```python
from build123d import *

# Parameters (mm, degrees)
BOSS_EXTRUDE1_DEPTH      = 7
EXTRUDE_THIN2_DEPTH      = 15
FILLET1_R                = 7
SKETCH5_W                = 15
SKETCH5_H                = 25
BOSS_EXTRUDE2_DEPTH      = 8
CUT_EXTRUDE2_DEPTH       = 42.641325627
LPATTERN1_COUNT          = 2
LPATTERN1_PITCH          = 26
CHAMFER3_SIZE            = 7
SKETCH9_W                = 15
SKETCH9_H                = 7
BOSS_EXTRUDE3_DEPTH      = 15
BOSS_EXTRUDE4_DEPTH      = 2
BOSS_EXTRUDE4_DEPTH_BACK = 9.9
SKETCH13_W               = 8
SKETCH13_H               = 2
BOSS_EXTRUDE6_DEPTH      = 6
CHAMFER6_SIZE            = 23.744712882
CHAMFER6_SIZE_2          = 13.5
CHAMFER7_SIZE            = 3
SKETCH14_R               = 1.5
CUT_EXTRUDE3_DEPTH       = 15
SKETCH15_W               = 15
SKETCH15_H               = 8.5
CUT_EXTRUDE4_DEPTH       = 6
CHAMFER8_SIZE            = 8
SKETCH16_W               = 3
SKETCH16_H               = 20
CUT_EXTRUDE5_DEPTH       = 54.176035971


with BuildPart() as part:
    # Sketch1 → Boss-Extrude1 (new body)
    with BuildSketch(Plane.XY):
        with BuildLine():
            Line((0, 25), (-20, 25))
            Line((-20, 25), (-20, -25))
            Line((-20, -25), (25, -25))
            Line((25, -25), (25, 0))
            ThreePointArc((25, 0), (17.67766953, 17.67766953), (0, 25))
        make_face()
    extrude(amount=BOSS_EXTRUDE1_DEPTH)

    # Sketch3 → Extrude-Thin2 (add)
    with BuildSketch(Plane.XY.offset(7)):
        with BuildLine():
            Line((25, -25), (25, 0))
            ThreePointArc((25, 0), (17.67766953, 17.67766953), (0, 25))
            Line((0, 25), (-20, 25))
            Line((-20, 25), (-20, 21))
            Line((-20, 21), (0, 21))
            ThreePointArc((0, 21), (14.849242405, 14.849242405), (21, 0))
            Line((21, 0), (21, -25))
            Line((21, -25), (25, -25))
        make_face()
    extrude(amount=EXTRUDE_THIN2_DEPTH)

    # Fillet1
    fillet1_edges = [part.edges().sort_by_distance(p)[0] for p in [
        (21, -12.5, 7),
        (14.849242405, 14.849242405, 7),
        (-10, 21, 7),
    ]]
    fillet(fillet1_edges, radius=FILLET1_R)

    # Sketch5 → Boss-Extrude2 (add)
    with BuildSketch(Plane(origin=(25, 0, 0), x_dir=(0, 0, -1), z_dir=(1, 0, 0))):
        with Locations((7.5, -12.5)):
            Rectangle(SKETCH5_W, SKETCH5_H)
    extrude(amount=-BOSS_EXTRUDE2_DEPTH)

    # Sketch8 → Cut-Extrude2 (cut, through all)
    with BuildSketch(Plane.XY.offset(7)):
        with BuildLine():
            Line((-14, -15), (-2, -15))
            ThreePointArc((-2, -15), (0, -17), (-2, -19))
            Line((-2, -19), (-14, -19))
            ThreePointArc((-14, -19), (-16, -17), (-14, -15))
        make_face()
    cut_extrude2 = extrude(amount=-CUT_EXTRUDE2_DEPTH, mode=Mode.SUBTRACT)

    # LPattern1: Cut-Extrude2 ×2
    with Locations(*[(0, i * LPATTERN1_PITCH, 0) for i in range(1, LPATTERN1_COUNT)]):
        add(cut_extrude2, mode=Mode.SUBTRACT)

    # Chamfer3
    chamfer3_edges = [part.edges().sort_by_distance(p)[0] for p in [
        (25, -12.5, -15),
    ]]
    chamfer(chamfer3_edges, length=CHAMFER3_SIZE)

    # Sketch9 → Boss-Extrude3 (add)
    with BuildSketch(Plane.ZY.offset(-17)):
        with Locations((-7.5, -3.5)):
            Rectangle(SKETCH9_W, SKETCH9_H)
    extrude(amount=BOSS_EXTRUDE3_DEPTH)

    # Sketch10 → Boss-Extrude4 (add, two sides: drawn at the far end of the back side and taken through both)
    with BuildSketch(Plane.XZ.offset(7).offset(-BOSS_EXTRUDE4_DEPTH_BACK)):
        Polygon((2, -15), (-6.970562748, -15), (-12.627416998, -9.343145751), (-16.870057685, -13.585786438), (-20, -10.455844123), (-20, 0), (17, 0), (17, -15), align=None)
        Polygon((-4.849242405, -10.050252532), (-9.091883092, -5.807611845), (-6.970562748, -3.686291501), (-2.727922061, -7.928932188), align=None, mode=Mode.SUBTRACT)
    extrude(amount=BOSS_EXTRUDE4_DEPTH + BOSS_EXTRUDE4_DEPTH_BACK)

    # Sketch13 → Boss-Extrude6 (add)
    with BuildSketch(Plane(origin=(-10.985281374, 0, -10.985281374), x_dir=(-0.7071067811865478, 0, 0.7071067811865472), z_dir=(-0.7071067811865472, 0, -0.7071067811865478))):
        with Locations((-1.67766953, 1.9)):
            Rectangle(SKETCH13_W, SKETCH13_H)
        with Locations((-1.67766953, -8)):
            Rectangle(SKETCH13_W, SKETCH13_H)
    extrude(amount=BOSS_EXTRUDE6_DEPTH)

    # Chamfer6
    # the kernel refuses this chamfer: 23.744712882, 13.5 mm, written as the material it adds along each edge
    with BuildSketch(Plane(origin=(-6.970562748, -9, -15), x_dir=(-0.7145740403020574, 0, -0.6995598194053126), z_dir=(0, 1, 0))) as chamfer6_piece_1_section:
        Polygon((CHAMFER6_SIZE * 0.999943641689, -CHAMFER6_SIZE * 0.0106166574102), (-CHAMFER6_SIZE_2 * 0.714574040302, -CHAMFER6_SIZE_2 * 0.699559819405), (0, 0), align=None)
    chamfer6_piece_1 = extrude(amount=2, mode=Mode.PRIVATE)
    chamfer6_piece_1 = split(chamfer6_piece_1, bisect_by=Plane(origin=(-9.095447466, -8, -21.360396657), z_dir=(0.7071067811865476, 0, 0.7071067811865476)), keep=Keep.TOP, mode=Mode.PRIVATE)
    add(chamfer6_piece_1)
    with BuildSketch(Plane(origin=(-6.970562748, -70.647744863, -15), x_dir=(-0.7145740403020574, 0, -0.6995598194053126), z_dir=(0, 1, 0))) as chamfer6_piece_2_section:
        Polygon((CHAMFER6_SIZE * 0.999943641689, -CHAMFER6_SIZE * 0.0106166574102), (-CHAMFER6_SIZE_2 * 0.714574040302, -CHAMFER6_SIZE_2 * 0.699559819405), (0, 0), align=None)
    chamfer6_piece_2 = extrude(amount=125.295489727, mode=Mode.PRIVATE)
    chamfer6_piece_2 = split(chamfer6_piece_2, bisect_by=Plane(origin=(-6.871868761, 2.9, -19.136817952), z_dir=(0, -1, 0)), keep=Keep.TOP, mode=Mode.PRIVATE)
    chamfer6_piece_2 = split(chamfer6_piece_2, bisect_by=Plane(origin=(-6.871868761, 0.9, -19.136817952), z_dir=(0, 1, 0)), keep=Keep.TOP, mode=Mode.PRIVATE)
    chamfer6_piece_2 = split(chamfer6_piece_2, bisect_by=Plane(origin=(-9.095447466, 1.9, -21.360396657), z_dir=(0.7071067811865476, 0, 0.7071067811865476)), keep=Keep.TOP, mode=Mode.PRIVATE)
    add(chamfer6_piece_2)
    with BuildSketch(Plane(origin=(-6.970562748, -60.747744863, -15), x_dir=(-0.7145740403020574, 0, -0.6995598194053126), z_dir=(0, 1, 0))) as chamfer6_piece_3_section:
        Polygon((CHAMFER6_SIZE * 0.999943641689, -CHAMFER6_SIZE * 0.0106166574102), (-CHAMFER6_SIZE_2 * 0.714574040302, -CHAMFER6_SIZE_2 * 0.699559819405), (0, 0), align=None)
    chamfer6_piece_3 = extrude(amount=125.295489727, mode=Mode.PRIVATE)
    chamfer6_piece_3 = split(chamfer6_piece_3, bisect_by=Plane(origin=(-6.871868761, -7, -19.136817952), z_dir=(0, -1, 0)), keep=Keep.TOP, mode=Mode.PRIVATE)
    chamfer6_piece_3 = split(chamfer6_piece_3, bisect_by=Plane(origin=(-9.095447466, -8, -21.360396657), z_dir=(0.7071067811865476, 0, 0.7071067811865476)), keep=Keep.TOP, mode=Mode.PRIVATE)
    chamfer6_piece_3 = split(chamfer6_piece_3, bisect_by=Plane(origin=(-6.871868761, -9, -19.136817952), z_dir=(0, 1, 0)), keep=Keep.TOP, mode=Mode.PRIVATE)
    add(chamfer6_piece_3)
    with BuildSketch(Plane(origin=(-6.970562748, 0.9, -15), x_dir=(-0.7145740403020574, 0, -0.6995598194053126), z_dir=(0, 1, 0))) as chamfer6_piece_4_section:
        Polygon((CHAMFER6_SIZE * 0.999943641689, -CHAMFER6_SIZE * 0.0106166574102), (-CHAMFER6_SIZE_2 * 0.714574040302, -CHAMFER6_SIZE_2 * 0.699559819405), (0, 0), align=None)
    chamfer6_piece_4 = extrude(amount=2, mode=Mode.PRIVATE)
    chamfer6_piece_4 = split(chamfer6_piece_4, bisect_by=Plane(origin=(-9.095447466, 1.9, -21.360396657), z_dir=(0.7071067811865476, 0, 0.7071067811865476)), keep=Keep.TOP, mode=Mode.PRIVATE)
    add(chamfer6_piece_4)

    # Chamfer7
    chamfer7_edges = [part.edges().sort_by_distance(p)[0] for p in [
        (-1.5, 2.9, 0),
        (17, -9, -7.5),
        (17, -17, 0),
        (-1.5, -9, 0),
    ]]
    chamfer(chamfer7_edges, length=CHAMFER7_SIZE)

    # Sketch14 → Cut-Extrude3 (cut)
    with BuildSketch(Plane(origin=(-10.985281374, 0, -10.985281374), x_dir=(-0.7071067811865478, 0, 0.7071067811865472), z_dir=(-0.7071067811865472, 0, -0.7071067811865478))):
        with Locations((-0.67766953, -3.05)):
            Circle(SKETCH14_R)
    extrude(amount=-CUT_EXTRUDE3_DEPTH, mode=Mode.SUBTRACT)

    # Sketch15 → Cut-Extrude4 (cut)
    with BuildSketch(Plane(origin=(-15.227922061, 0, -15.227922061), x_dir=(-0.7071067811865475, 0, 0.7071067811865477), z_dir=(-0.7071067811865477, 0, -0.7071067811865475))):
        with Locations((-4.87766953, -3.05)):
            Rectangle(SKETCH15_W, SKETCH15_H)
    extrude(amount=-CUT_EXTRUDE4_DEPTH, mode=Mode.SUBTRACT)

    # Chamfer8
    # the kernel refuses this chamfer: 8 mm, written as the material it adds along each edge
    with BuildSketch(Plane(origin=(17, 0, 0), x_dir=(0.9996219169112968, -0.02749587661058649, 0), z_dir=(0, 0, -1))) as chamfer8_piece_1_section:
        Polygon((CHAMFER8_SIZE * 0.999621916911, -CHAMFER8_SIZE * 0.0274958766106), (-CHAMFER8_SIZE * 0.0274958766106, -CHAMFER8_SIZE * 0.999621916911), (0, 0), align=None)
    chamfer8_piece_1 = extrude(amount=15, mode=Mode.PRIVATE)
    chamfer8_piece_1 = split(chamfer8_piece_1, bisect_by=Plane(origin=(25, 1.068527792, -2.415736104), z_dir=(-1, 0, 0)), keep=Keep.TOP, mode=Mode.PRIVATE)
    chamfer8_piece_1 = split(chamfer8_piece_1, bisect_by=Plane(origin=(20.463014023, 2.9, -2.415736104), z_dir=(0, -1, 0)), keep=Keep.TOP, mode=Mode.PRIVATE)
    chamfer8_piece_1 = split(chamfer8_piece_1, bisect_by=Plane(origin=(20.463014023, 2.276395844, -3.623604156), z_dir=(0, -0.7071067811865476, 0.7071067811865476)), keep=Keep.TOP, mode=Mode.PRIVATE)
    add(chamfer8_piece_1)
    with BuildSketch(Plane(origin=(17, 0, 20.573463904), x_dir=(0.9996219169112968, -0.02749587661058651, 0), z_dir=(0, 0, -1))) as chamfer8_piece_2_section:
        Polygon((CHAMFER8_SIZE * 0.999621916911, -CHAMFER8_SIZE * 0.0274958766106), (-CHAMFER8_SIZE * 0.0274958766106, -CHAMFER8_SIZE * 0.999621916911), (0, 0), align=None)
    chamfer8_piece_2 = extrude(amount=35.573463904, mode=Mode.PRIVATE)
    chamfer8_piece_2 = split(chamfer8_piece_2, bisect_by=Plane(origin=(17.28092154, 7.132229333, 0), z_dir=(0, 0, 1)), keep=Keep.TOP, mode=Mode.PRIVATE)
    chamfer8_piece_2 = split(chamfer8_piece_2, bisect_by=Plane(origin=(17.28092154, 6.824172, 0.924172), z_dir=(0, 0.7071067811865476, -0.7071067811865476)), keep=Keep.TOP, mode=Mode.PRIVATE)
    add(chamfer8_piece_2)
    with BuildSketch(Plane(origin=(17, 0, 0), x_dir=(0.9996219169112968, -0.02749587661058649, 0), z_dir=(0, 0, -1))) as chamfer8_piece_3_section:
        Polygon((CHAMFER8_SIZE * 0.999621916911, -CHAMFER8_SIZE * 0.0274958766106), (-CHAMFER8_SIZE * 0.0274958766106, -CHAMFER8_SIZE * 0.999621916911), (0, 0), align=None)
    chamfer8_piece_3 = extrude(amount=15, mode=Mode.PRIVATE)
    chamfer8_piece_3 = split(chamfer8_piece_3, bisect_by=Plane(origin=(19.029775324, 2.9, -1.05711343), z_dir=(0, 1, 0)), keep=Keep.TOP, mode=Mode.PRIVATE)
    chamfer8_piece_3 = split(chamfer8_piece_3, bisect_by=Plane(origin=(19.029775324, 4.314329856, -1.585670144), z_dir=(0, -0.7071067811865476, 0.7071067811865476)), keep=Keep.TOP, mode=Mode.PRIVATE)
    add(chamfer8_piece_3)
    with BuildSketch(Plane(origin=(17, 0, 0), x_dir=(0.9996219169112968, -0.02749587661058649, 0), z_dir=(0, 0, -1))) as chamfer8_piece_4_section:
        Polygon((CHAMFER8_SIZE * 0.999621916911, -CHAMFER8_SIZE * 0.0274958766106), (-CHAMFER8_SIZE * 0.0274958766106, -CHAMFER8_SIZE * 0.999621916911), (0, 0), align=None)
    chamfer8_piece_4 = extrude(amount=15, mode=Mode.PRIVATE)
    chamfer8_piece_4 = split(chamfer8_piece_4, bisect_by=Plane(origin=(21.997895662, 1.393550415, -11.002104338), z_dir=(-0.7071067811865476, 0, 0.7071067811865476)), keep=Keep.TOP, mode=Mode.PRIVATE)
    chamfer8_piece_4 = split(chamfer8_piece_4, bisect_by=Plane(origin=(25, 1.393550415, -8.795226249), z_dir=(-1, 0, 0)), keep=Keep.TOP, mode=Mode.PRIVATE)
    chamfer8_piece_4 = split(chamfer8_piece_4, bisect_by=Plane(origin=(19.791017572, 2.9, -8.795226249), z_dir=(0, -1, 0)), keep=Keep.TOP, mode=Mode.PRIVATE)
    chamfer8_piece_4 = split(chamfer8_piece_4, bisect_by=Plane(origin=(19.791017572, -0.750837917, -6.650837917), z_dir=(0, 0.7071067811865476, -0.7071067811865476)), keep=Keep.TOP, mode=Mode.PRIVATE)
    add(chamfer8_piece_4)

    # Sketch16 → Cut-Extrude5 (cut, through all)
    with BuildSketch(Plane.ZY.offset(-21)):
        with Locations((17.5, -2)):
            Rectangle(SKETCH16_W, SKETCH16_H)
    extrude(amount=-CUT_EXTRUDE5_DEPTH, mode=Mode.SUBTRACT)


solid = part.part
```
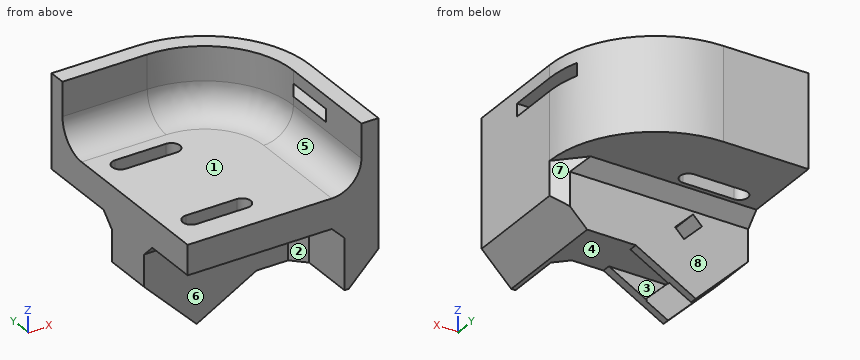
The model under review builds one solid part; all positions refer to its coordinate system, in mm. Face numbers are marked on the shaded views. A direction names the side the tool comes from. Coordinates: 2 decimals unless noted, no trailing zeros. Write each loop counter-clockwise with the first axis right and the second up, starting at its lowest first coordinate (ties: lowest second). Pieces come first, ordered by that corner, then holes.
1) To check wall thickness, follow probe 1 along Z at (x, y) = (3, -2.5); probe 2 along X at (y, z) = (-2, -1); probe 3 along Y at (x, z) = (-3, -6.5). State the ranges of each line that lie inside material, in increasing order.
2) The part is to be moulded in two halves that separate along Y. For the marked faces 1, 2, 3 and 4, say which applies: pulls with the +Y half, pulls with the -Y half, needs draft (parallel to the pull), parting line crosses it, or undercut.
3) We need section A-A on y = -17. State the section outline as (x, z) points.
4) We need section C-C on x = -4. Count the separate pieces of the cut face and the enclosed holes in it, then the cut area to 3 significant figures.
5) Machinability: for the marked faces 5, 6, 7 and 8, which of the approach directions +Z, -Z, +X, -X, +Y, -Y give a long, thin tool a straight path to every point of the face, cutting with its end or side? Answer none if there is none.
6) Clearance check with flat-ended pins moving along their axes: pin 1 Ø15 at (x, z) = (-12.5, -19) entering from -Y; pin 2 Ø3.5 at (x, z) = (23, 17.5) entering from +Y; pin 3 Ø2 at (x, y) = (11, 16) entering from -Z; pin 4 Ø1.5 at (x, z) = (2.5, -18.5) entering from -Y. State where each tip first meets the part, or that it passes through.
7) We need section B-B on z = 2.5. State the section outline as (x, y) points.
8) We need section D-D on z = 9. State the section outline as (x, y) points, then the cut area to 3 significant figures.
Answer list:
1. probe 1: z = -15 to 7
1. probe 2: x = -20 to -1.56, 0.24 to 25
1. probe 3: y = -9 to 2.9
2. face 1: needs draft
2. face 2: pulls with the -Y half
2. face 3: undercut
2. face 4: undercut
3. outline: (-20, 0) - (-16, 0) - (-16, 7) - (-20, 7) - close; (0, 0) - (14, 0) - (17, -3) - (17, -15) - (18, -15) - (25, -8) - (25, 22) - (21, 22) - (21, 14) arc R7 cw to (14, 7) - (0, 7) - close
4. separate pieces: 4
4. enclosed holes: 0
4. area: 534 mm2
5. face 5: +Z, -X, -Y
5. face 6: -Z, -X, -Y
5. face 7: -Z, +X, +Y
5. face 8: -Z, +X, -X, +Y
6. pin 1: stops at y = -9
6. pin 2: stops at y = 13.17
6. pin 3: stops at z = 0
6. pin 4: passes through
7. outline: (-20, -25) - (25, -25) - (25, 0) arc R25 ccw to (0, 25) - (-20, 25) - close; hole (-14, -19) - (-2, -19) arc R2 ccw to (-2, -15) - (-14, -15) arc R2 ccw to start; hole (-14, 7) - (-2, 7) arc R2 ccw to (-2, 11) - (-14, 11) arc R2 ccw to start
8. outline: (-20, 18.9) - (0, 18.9) arc R18.9 cw to (18.9, 0) - (18.9, -25) - (25, -25) - (25, 0) arc R25 ccw to (0, 25) - (-20, 25) - close
8. area: 485 mm2
